The model under review builds one solid part; all positions refer to its coordinate system, in mm. Coordinates: 2 decimals unless noted, no trailing zeros. Order: outer loops, then holes, each group sorted by start corner. A loop starts at its lowest first (then second) coordinate and runs counter-clockwise, first axis right, second up. Notation, with made-up numbers: M -21,-33 L 8,-33 A12 cw 8,-15 Z; hole C 35,35.5 d8. An arc over 180 degrees is marked long. Answer in a Markdown table with one row per item.
from build123d import *

# Parameters (mm, degrees)
SKETCH1_W              = 123.825
SKETCH1_H              = 92.075
BOSS_EXTRUDE2_DEPTH    = 4.7625
SKETCH2_R              = 11.1125
SKETCH2_R_2            = 14.2875
CUT_EXTRUDE1_DEPTH     = 5.7625
F_10_CLEARANCE_HOLE1_D = 5.1054
SKETCH8_R              = 14.2875
CUT_EXTRUDE3_DEPTH     = 5.7625
SKETCH9_R              = 14.2875
SKETCH9_R_2            = 11.1125
BOSS_EXTRUDE3_DEPTH    = 4.7625
BOSS_EXTRUDE4_DEPTH    = 4.7625
F_10_CLEARANCE_HOLE2_D = 5.1054


with BuildPart() as part:
    # Sketch1 → Boss-Extrude2 (new body)
    with BuildSketch(Plane(origin=(0, 0, 0), x_dir=(0, 0, -1), z_dir=(1, 0, 0))):
        with Locations((61.9125, 46.0375)):
            Rectangle(SKETCH1_W, SKETCH1_H)
    extrude(amount=BOSS_EXTRUDE2_DEPTH)

    # Sketch2 → Cut-Extrude1 (cut, through all)
    with BuildSketch(Plane(origin=(4.7625, 0, 0), x_dir=(0, 0, -1), z_dir=(1, 0, 0))):
        with Locations((66.2432, 57.15)):
            Circle(SKETCH2_R)
        with Locations((31.75, 57.15)):
            Circle(SKETCH2_R)
        with Locations((90.633575625, 32.759624375)):
            Circle(SKETCH2_R_2)
    extrude(amount=-CUT_EXTRUDE1_DEPTH, mode=Mode.SUBTRACT)

    # #10 Clearance Hole1 (through all)
    with Locations(Plane(origin=(4.7625, 0, 0), x_dir=(0, 0, -1), z_dir=(1, 0, 0))):
        with Locations((9.525, 84.829624375), (111.125, 61.334624375), (9.525, 32.759624375), (111.125, 16.884624375)):
            Hole(F_10_CLEARANCE_HOLE1_D / 2)

    # Sketch8 → Cut-Extrude3 (cut, through all)
    with BuildSketch(Plane(origin=(4.7625, 0, 0), x_dir=(0, 0, -1), z_dir=(1, 0, 0))):
        with Locations((31.75, 57.15)):
            Circle(SKETCH8_R)
    extrude(amount=-CUT_EXTRUDE3_DEPTH, mode=Mode.SUBTRACT)

    # Sketch9 → Boss-Extrude3 (add)
    with BuildSketch(Plane(origin=(4.7625, 0, 0), x_dir=(0, 0, -1), z_dir=(1, 0, 0))):
        with Locations((90.633575625, 32.759624375)):
            Circle(SKETCH9_R)
        with Locations((90.633575625, 32.759624375)):
            Circle(SKETCH9_R_2, mode=Mode.SUBTRACT)
    extrude(amount=-BOSS_EXTRUDE3_DEPTH)

    # Sketch11 → Boss-Extrude4 (add)
    with BuildSketch(Plane.ZY):
        with BuildLine():
            Line((-132.034871939, -14.015128061), (-118.019743879, 0))
            Line((-118.019743879, 0), (-123.825, 0))
            Line((-123.825, 0), (-123.825, 12.155256121))
            Line((-123.825, 12.155256121), (-141.015128061, -5.034871939))
            ThreePointArc((-141.015128061, -5.034871939), (-141.015128061, -14.015128061), (-132.034871939, -14.015128061))
        make_face()
        with BuildLine():
            Line((-139.7, 92.925738686), (-123.825, 83.760303163))
            Line((-123.825, 83.760303163), (-123.825, 92.075))
            Line((-123.825, 92.075), (-112.826477372, 92.075))
            Line((-112.826477372, 92.075), (-133.35, 103.924261314))
            ThreePointArc((-133.35, 103.924261314), (-142.024261314, 101.6), (-139.7, 92.925738686))
        make_face()
        with BuildLine():
            Line((-15.875, -9.525), (-15.875, 0))
            Line((-15.875, 0), (-3.175, 0))
            Line((-3.175, 0), (-3.175, -9.525))
            ThreePointArc((-3.175, -9.525), (-9.525, -15.875), (-15.875, -9.525))
        make_face()
        with BuildLine():
            Line((-15.875, 98.425), (-15.875, 92.075))
            Line((-15.875, 92.075), (-3.175, 92.075))
            Line((-3.175, 92.075), (-3.175, 98.425))
            ThreePointArc((-3.175, 98.425), (-9.525, 104.775), (-15.875, 98.425))
        make_face()
    extrude(amount=-BOSS_EXTRUDE4_DEPTH)

    # #10 Clearance Hole2 (through all)
    with Locations(Plane.ZY):
        with Locations((-136.525, -9.525), (-136.525, 98.425), (-9.525, 98.425), (-9.525, -9.525)):
            Hole(F_10_CLEARANCE_HOLE2_D / 2)


solid = part.part
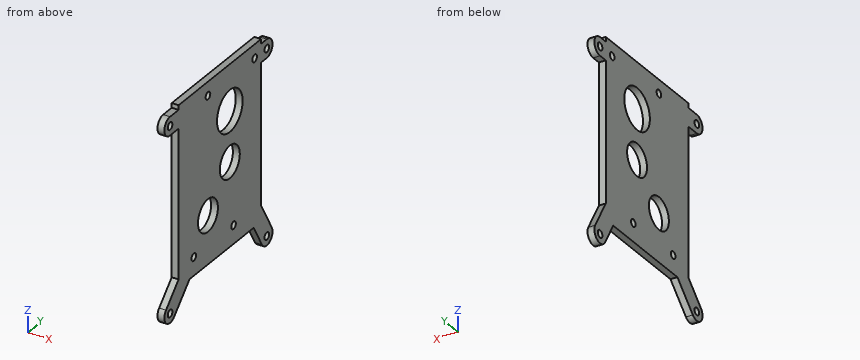
(1) To check wall thickness, follow line 1 (Y direction, x = 4.55, z = -91) (3 decimals); line 2 (Z direction, x = 1.8, y = -11); line 3 (Y direction, x = 1.5, z = -91.5) (3 decimals). State the ranges of each line that lie inside material, in increasing order. Write a range as [from, to].
Report:
| item | result |
|---|---|
| line 1 | [0, 21.653], [43.866, 92.075] |
| line 2 | [-142.7, -138.61], [-134.44, -129.02], [-15.7, -11.61], [-7.44, -3.35] |
| line 3 | [0, 21.681], [43.838, 92.075] |
(2) Insertion check: P1, Ø1.4, axis at x = 2, z = -75, coming from the -Y side; P2, Ø3, axis at y = 61.33, z = -111.12, coming from the +X side; P3, Ø1, axis at x = 2.5, z = -1, coming from the +Y side (3 decimals); P4, Ø1.4, axis at x = 2.5, y = 95.5, coming from the +Z side (3 decimals). Each pin has a flat end and moves straight along its axis. Give the tip position at first contact, or say it passes through.
Report:
| item | result |
|---|---|
| P1 | y = 0 |
| P2 | through |
| P3 | y = 92.075 |
| P4 | z = -3.175 |
(3) Take a section at B-B (y = 57.15). Write out the cut boundary in (x, z) (1 decimal).
Report:
| item | result |
|---|---|
| outline | M 0,-123.8 L 4.8,-123.8 L 4.8,-77.4 L 0,-77.4 Z; M 0,-55.1 L 4.8,-55.1 L 4.8,-46 L 0,-46 Z; M 0,-17.5 L 4.8,-17.5 L 4.8,0 L 0,0 Z |
(4) Take a section at C-C (y = 28.5). Write out the cut boundary in (x, z) (1 decimal), then the cut area to 3 significant figures.
Report:
| item | result |
|---|---|
| outline | M 0,-123.8 L 4.8,-123.8 L 4.8,-100.9 L 0,-100.9 Z; M 0,-80.4 L 4.8,-80.4 L 4.8,0 L 0,0 Z |
| area | 492 mm^2 |
(5) Take a section at D-D (x = 2.55). State how many separate pieces and enclosed holes the cut face has, then the cut area to 3 significant figures.
Report:
| item | result |
|---|---|
| separate pieces | 1 |
| enclosed holes | 11 |
| area | 10,700 mm^2 |
(6) Take a section at A-A (z = -31.75). Write out the cut boundary in (x, y) (1 decimal), then the cut area to 3 significant figures.
Report:
| item | result |
|---|---|
| outline | M 0,0 L 4.8,0 L 4.8,42.9 L 0,42.9 Z; M 0,71.4 L 4.8,71.4 L 4.8,92.1 L 0,92.1 Z |
| area | 302 mm^2 |
